For this review, take the finished solid that the model builds, in its own axes (mm). A direction names the side the tool comes from. Round coordinates to 2 decimals unless told otherwise and drop trailing zeros. Order: outer loops, then holes, each group sorted by start corner. A loop starts at its lowest first (then second) coordinate and runs counter-clockwise, first axis right, second up. Notation, with made-up numbers: (44.25, 52.25) -> (51.25, 52.25) arc R14 ccw to (51.25, 62.25) -> close; hole circle Ø3 at (-21.5, 82.25). An arc over 180 degrees is marked (long way). Use a Markdown table: item, result. Add a question column.
1) Clearance check with a flat-ended pin moving along its axis: P1, Ø1, axis at x = -2.5, z = 0.5, coming from the +Y side. State where the tip first meets the part, or that it passes through.
2) Draft analysis for pull direction Y (two halves, no side actions). For faces 4 (the face through (3.233, -1.341, 0.74)), 5 (the face through (1.6, -1.6, 1.8)), 6 (the face through (1.43, -1.54, 1.65)), state which applies: pulls with the +Y half, pulls with the -Y half, needs draft (parallel to the pull), parting line crosses it, or undercut.
3) Consider section B-B (y = 0.9). State the section outline as (x, z) points, plus the area to 3 significant figures.
4) Wall thickness on line 1 along Z through (x, y) = (-0.25, -2.5); line 2 along Y through (x, z) = (2.75, 0.4); line 3 along Y through (x, z) = (0.75, 0.8): over which ranges is each line inside the solid? List them lowest first. Write a range as [from, to].
5) Consider section A-A (x = 1.25). State the section outline as (y, z) points.
6) Consider section D-D (x = 0). State the section outline as (y, z) points, plus the area to 3 significant figures.
7) Machinability: for faces 1 (the face through (0, 0, 1.5)), 2 (the face through (0, 0, 0)), 3 (the face through (1.74, -1.93, 1.65)), which of the approach directions +Z, -Z, +X, -X, +Y, -Y give a long, thin tool a straight path to every point of the face, cutting with its end or side? Answer none if there is none.
8) Consider section C-C (z = 0.35). State the section outline as (x, y) points, plus the area to 3 significant figures.
```python
from build123d import *

# Parameters (mm, degrees)
F0_R     = 3.5
F1_DEPTH = 1.5
F2_R     = 0.35
F3_DEPTH = 1.8


with BuildPart() as f1:
    # F0 (on Top) → F1 (new body)
    with BuildSketch(Plane.XY):
        Circle(F0_R)
    extrude(amount=F1_DEPTH)

    # F2 (on Top) → F3 (join)
    with BuildSketch(Plane.XY):
        with Locations((-1.3, 0.9)):
            Circle(F2_R)
        with Locations((1.3, 0.9)):
            Circle(F2_R)
        with BuildLine():
            Line((0.183027, -2.092009), (0.226605, -2.590106))
            ThreePointArc((0.226605, -2.590106), (1.756535, -1.916921), (2.5605, -0.451485))
            Line((2.5605, -0.451485), (2.068096, -0.364661))
            ThreePointArc((2.068096, -0.364661), (1.418739, -1.548282), (0.183027, -2.092009))
        make_face()
    extrude(amount=F3_DEPTH)


solid = f1.part
```
Results list:
| question | item | result |
|---|---|---|
| 1 | P1 | y = 2.87 |
| 2 | face 4 | parting line crosses it |
| 2 | face 5 | needs draft |
| 2 | face 6 | undercut |
| 3 | outline | (-3.38, 0) -> (3.38, 0) -> (3.38, 1.5) -> (1.65, 1.5) -> (1.65, 1.8) -> (0.95, 1.8) -> (0.95, 1.5) -> (-0.95, 1.5) -> (-0.95, 1.8) -> (-1.65, 1.8) -> (-1.65, 1.5) -> (-3.38, 1.5) -> close |
| 3 | area | 10.6 mm2 |
| 4 | line 1 | [0, 1.5] |
| 4 | line 2 | [-2.17, 2.17] |
| 4 | line 3 | [-3.42, 3.42] |
| 5 | outline | (-3.27, 0) -> (3.27, 0) -> (3.27, 1.5) -> (1.25, 1.5) -> (1.25, 1.8) -> (0.55, 1.8) -> (0.55, 1.5) -> (-1.69, 1.5) -> (-1.69, 1.8) -> (-2.28, 1.8) -> (-2.28, 1.5) -> (-3.27, 1.5) -> close |
| 6 | outline | (-3.5, 0) -> (3.5, 0) -> (3.5, 1.5) -> (-3.5, 1.5) -> close |
| 6 | area | 10.5 mm2 |
| 7 | face 1 | +Z |
| 7 | face 2 | -Z, +X, -X, +Y, -Y |
| 7 | face 3 | +Z, +X, -Y |
| 8 | outline | circle Ø7 at (0, 0) |
| 8 | area | 38.5 mm2 |
